```python
from build123d import *

# Parameters (mm, degrees)
SKETCH2_W                       = 12.7
SKETCH2_H                       = 22.225
BOSS_EXTRUDE1_DEPTH             = 6.35
BOSS_EXTRUDE1_2_DEPTH           = 6.35
SKETCH2_W_2                     = 19.05
BOSS_EXTRUDE1_3_DEPTH           = 6.35
SKETCH2_3_W                     = 6.35
SKETCH2_3_H                     = 22.225
BOSS_EXTRUDE2_DEPTH             = 31.75
SKETCH3_R                       = 3.175
CUT_EXTRUDE1_DEPTH              = 59.973007597
F_1_4_0_25_DIAMETER_HOLE1_D     = 6.35
F_1_4_0_25_DIAMETER_HOLE1_DEPTH = 25.4
F_1_4_0_25_DIAMETER_HOLE1_TIP   = 1.907732465
FILLET1_R                       = 8.255


with BuildPart() as part:
    # Sketch2 → Boss-Extrude1 (new body)
    with BuildSketch(Plane(origin=(0, 0, 0), x_dir=(1, 0, 0), z_dir=(0, 1, 0))):
        with Locations((6.35, 11.1125)):
            Rectangle(SKETCH2_W, SKETCH2_H)
    extrude(amount=BOSS_EXTRUDE1_DEPTH)



with BuildPart() as body_2:
    # Sketch2 → Boss-Extrude1 2 (new body)
    with BuildSketch(Plane(origin=(0, 0, 0), x_dir=(1, 0, 0), z_dir=(0, 1, 0))):
        with Locations((50.8, 11.1125)):
            Rectangle(SKETCH2_W, SKETCH2_H)
    extrude(amount=BOSS_EXTRUDE1_2_DEPTH)


with BuildPart() as body_3:
    # Sketch2 → Boss-Extrude1 3 (new body)
    with BuildSketch(Plane(origin=(0, 0, 0), x_dir=(1, 0, 0), z_dir=(0, 1, 0))):
        with Locations((28.575, 11.1125)):
            Rectangle(SKETCH2_W_2, SKETCH2_H)
    extrude(amount=BOSS_EXTRUDE1_3_DEPTH)


with BuildPart() as part_1:
    add(part.part)

    add(body_2.part)  # Boss-Extrude2 merges body 2

    add(body_3.part)  # Boss-Extrude2 merges body 3
    # Sketch2_3 → Boss-Extrude2 (add)
    with BuildSketch(Plane(origin=(0, 0, 0), x_dir=(1, 0, 0), z_dir=(0, 1, 0))):
        with Locations((15.875, 11.1125)):
            Rectangle(SKETCH2_3_W, SKETCH2_3_H)
        with Locations((41.275, 11.1125)):
            Rectangle(SKETCH2_3_W, SKETCH2_3_H)
    extrude(amount=BOSS_EXTRUDE2_DEPTH)

    # Sketch3 → Cut-Extrude1 (cut, through all)
    with BuildSketch(Plane.ZY.offset(-12.7)):
        with Locations(Location((-11.1125, 25.4, 0), (0, 0, 180))):
            Circle(SKETCH3_R)
    extrude(amount=-CUT_EXTRUDE1_DEPTH, mode=Mode.SUBTRACT)

    # 1_4 _0.25_ Diameter Hole1
    with Locations(Plane(origin=(6.35, 6.35, -11.1125), x_dir=(0, 0, 1), z_dir=(0, 1, 0))):
        with Locations((0, 0), (0, 22.225), (0, 44.45)):
            Hole(F_1_4_0_25_DIAMETER_HOLE1_D / 2, depth=F_1_4_0_25_DIAMETER_HOLE1_DEPTH)
            with Locations((0, 0, -(F_1_4_0_25_DIAMETER_HOLE1_DEPTH + F_1_4_0_25_DIAMETER_HOLE1_TIP / 2))):  # 118° drill point
                Cone(0, F_1_4_0_25_DIAMETER_HOLE1_D / 2, F_1_4_0_25_DIAMETER_HOLE1_TIP, mode=Mode.SUBTRACT)

    # Fillet1
    fillet1_edges = [part_1.edges().sort_by_distance(p)[0] for p in [
        (15.875, 31.75, -22.225),
        (41.275, 31.75, -22.225),
        (41.275, 31.75, 0),
        (15.875, 31.75, 0),
    ]]
    fillet(fillet1_edges, radius=FILLET1_R)


solid = part_1.part
```
Read the model definition and answer for the solid it produces. Units are mm, in the model's axes. A direction names the side the tool comes from. Round coordinates to 2 decimals unless told otherwise and drop trailing zeros. Write each loop counter-clockwise with the first axis right and the second up, starting at its lowest first coordinate (ties: lowest second). Pieces come first, ordered by that corner, then holes. Notation, with made-up numbers: (31, -22.75) -> (56, -22.75) arc R21 ccw to (56, -6.75) -> close; hole circle Ø6 at (21.5, -35.75). An arc over 180 degrees is marked (long way). Answer in a Markdown table with one row per item. Add a question column.
1) Determine the mould class of faces 6 (the face through (16, 31.75, -11)), 7 (the face through (15.919, 29.268, -2.354)), 8 (the face through (25.476, 3.131, -10.424)), 9 (the face through (41.23, 22.25, -10.7)) for opening direction Z: pulls with the +Z half, pulls with the -Z half, needs draft (parallel to the pull), parting line crosses it, or undercut.
2) Which of the six approach directions +Z, -Z, +X, -X, +Y, -Y give full straight-line access (tool end or side, diameter ignored) to faces 1 (the face through (28, 0, -16)), 2 (the face through (15.92, 29.27, -19.87)), 3 (the face through (12.7, 19, -11)), 4 (the face through (26, 6.35, -14)), 5 (the face through (44.45, 19, -11))?
3) Find section B-B, the plane y = 8.5. Determine the outline of the cut face in (x, z) (3 decimals).
4) Find section D-D, the plane y = 25.4. Determine the outline of the cut face in (x, z), and give its area (3 significant figures).
5) Given P1, Ø6.5, axis at y = 16, z = -15, coming from the +X side; P2, Ø4, axis at y = 25.4, z = -11.11, coming from the +X side; P3, Ø11, axis at y = 19.5, z = -8, coming from the -X side; P4, Ø1, axis at x = 24.5, z = -5, coming from the +Y side, each flat-ended and moving along its own axis, determine where each tip first touches the part or whether it passes through.
6) Consider line 1 (X direction, y = 7, z = -3.25); line 2 (X direction, y = 6, z = -9.75); line 3 (Y direction, x = 52, z = -7.75). Determine where each line is inside the solid, lowest interval first.
Findings below:
| question | item | result |
|---|---|---|
| 1 | face 6 | needs draft |
| 1 | face 7 | pulls with the +Z half |
| 1 | face 8 | undercut |
| 1 | face 9 | undercut |
| 2 | face 1 | +Z, -Z, +X, -X, -Y |
| 2 | face 2 | -Z, +X, -X, +Y |
| 2 | face 3 | +Z, -Z, -X, +Y |
| 2 | face 4 | +Z, -Z, +Y |
| 2 | face 5 | +Z, -Z, +X, +Y |
| 3 | outline | (12.7, -22.225) -> (19.05, -22.225) -> (19.05, 0) -> (12.7, 0) -> close; (38.1, -22.225) -> (44.45, -22.225) -> (44.45, 0) -> (38.1, 0) -> close |
| 4 | outline | (12.7, -22) -> (19.05, -22) -> (19.05, -14.29) -> (12.7, -14.29) -> close; (12.7, -7.94) -> (19.05, -7.94) -> (19.05, -0.22) -> (12.7, -0.22) -> close; (38.1, -22) -> (44.45, -22) -> (44.45, -14.29) -> (38.1, -14.29) -> close; (38.1, -7.94) -> (44.45, -7.94) -> (44.45, -0.22) -> (38.1, -0.22) -> close |
| 4 | area | 196 mm² |
| 5 | P1 | x = 44.45 |
| 5 | P2 | through |
| 5 | P3 | x = 12.7 |
| 5 | P4 | y = 6.35 |
| 6 | line 1 | 12.7 to 19.05, 38.1 to 44.45 |
| 6 | line 2 | 0 to 3.48, 9.22 to 25.71, 31.44 to 47.93, 53.67 to 57.15 |
| 6 | line 3 | 0 to 6.35 |
